```python
from build123d import *

# Parameters (mm, degrees)
SKETCH1_W           = 80
SKETCH1_H           = 40
BOSS_EXTRUDE1_DEPTH = 3
SKETCH2_R           = 2
SKETCH2_R_2         = 1
BOSS_EXTRUDE3_DEPTH = 10
LPATTERN1_COUNT     = 2
LPATTERN1_PITCH     = 20
SKETCH3_R           = 2
SKETCH3_R_2         = 1
BOSS_EXTRUDE4_DEPTH = 15
LPATTERN2_COUNT     = 2
LPATTERN2_PITCH     = 25


with BuildPart() as part:
    # Sketch1 → Boss-Extrude1 (new body)
    with BuildSketch(Plane.XY):
        Rectangle(SKETCH1_W, SKETCH1_H)
    extrude(amount=BOSS_EXTRUDE1_DEPTH)

    # Sketch2 → Boss-Extrude3 (add)
    with BuildSketch(Plane(origin=(0, 20, 0), x_dir=(1, 0, 0), z_dir=(0, 1, 0))):
        with Locations((-41.322875656, -1.5)):
            Circle(SKETCH2_R)
        with Locations(Location((-41.322875656, -1.5, 0), (0, 0, 270))):
            Circle(SKETCH2_R_2, mode=Mode.SUBTRACT)
    boss_extrude3 = extrude(amount=-BOSS_EXTRUDE3_DEPTH)

    # LPattern1: Boss-Extrude3 ×2
    with Locations(*[(0, -i * LPATTERN1_PITCH, 0) for i in range(1, LPATTERN1_COUNT)]):
        add(boss_extrude3)

    # Sketch3 → Boss-Extrude4 (add)
    with BuildSketch(Plane(origin=(0, 20, 0), x_dir=(1, 0, 0), z_dir=(0, 1, 0))):
        with Locations((41.322875656, -1.5)):
            Circle(SKETCH3_R)
        with Locations(Location((41.322875656, -1.5, 0), (0, 0, 270))):
            Circle(SKETCH3_R_2, mode=Mode.SUBTRACT)
    boss_extrude4 = extrude(amount=-BOSS_EXTRUDE4_DEPTH)

    # LPattern2: Boss-Extrude4 ×2
    with Locations(*[(0, -i * LPATTERN2_PITCH, 0) for i in range(1, LPATTERN2_COUNT)]):
        add(boss_extrude4)


solid = part.part
```
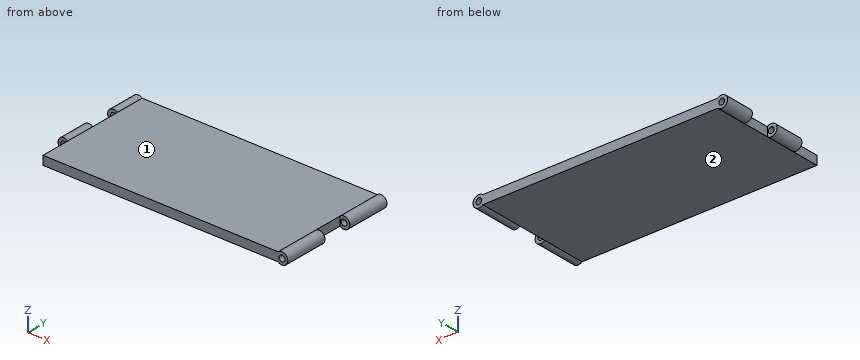
Geometry check sheet. Reference: the model listing, model coordinates, mm. Face numbers are marked on the shaded views. Give positions to 0.01 mm unless a question says otherwise; leave off trailing zeros. Write each loop counter-clockwise with the first axis right and the second up, starting at its lowest first coordinate (ties: lowest second). Pieces come first, ordered by that corner, then holes. Notation, with made-up numbers: (20.25, -36.5) -> (36.25, -36.5) arc R33 ccw to (36.25, -6.5) -> close; hole circle Ø6 at (42, 33.25). An arc over 180 degrees is marked (long way). One line per question, with ' | ' between items.
Item 1: Sectioned sample at C-C, the plane y = -16.5. Record the boundary of the cut face in (x, z), plus the area to 3 significant figures.
Determined:
outline: (-40, 0) -> (40, 0) arc R2 ccw (long way) to (40, 3) -> (-40, 3) -> close; hole circle Ø2 at (41.32, 1.5) | area: 248 mm^2
Item 2: Sectioned sample at A-A, the plane z = 1.5. State how many separate pieces and enclosed holes the cut face has, plus the area to 3 significant figures.
Determined:
separate pieces: 5 | enclosed holes: 0 | area: 3,270 mm^2
Item 3: Sectioned sample at B-B, the plane y = -7. Record the boundary of the cut face in (x, z), plus the area to 3 significant figures.
Determined:
outline: (-40, 0) -> (40, 0) arc R2 ccw (long way) to (40, 3) -> (-40, 3) arc R2 ccw (long way) to start; hole circle Ø2 at (-41.32, 1.5); hole circle Ø2 at (41.32, 1.5) | area: 256 mm^2
Item 4: Draft check along X on the marked faces 1 and 2. Enter one of: released by +X, released by -X, zero draft, split by the parting line, or undercut.
Determined:
face 1: undercut | face 2: undercut
Item 5: Sectioned sample at D-D, the plane x = 38.5. Record the boundary of the cut face in (y, z), plus the area to 3 significant figures.
Determined:
outline: (-20, 0) -> (20, 0) -> (20, 3) -> (-20, 3) -> close | area: 120 mm^2
Item 6: Scan lines: line 1 along X through (y, z) = (13.75, 1.5); line 2 along X through (y, z) = (-2.75, 1.5); line 3 along X through (y, z) = (-14.5, 1.5). Record each from-to range of solid material in increasing order.
Determined:
line 1: -43.32 to -42.32, -40.32 to 40.32, 42.32 to 43.32 | line 2: -43.32 to -42.32, -40.32 to 40 | line 3: -40 to 40.32, 42.32 to 43.32
Item 7: Depth check by flat-ended pin: pin 1 (1.5 mm diameter, centred on y = 4, z = 1, fed in from +X); pin 2 (20 mm diameter, centred on x = 9, y = -9.5, fed in from -Z); pin 3 (12 mm diameter, centred on x = 20.5, y = 5.5, fed in from +Z); pin 4 (1.8 mm diameter, centred on x = -41.32, z = 1.5, fed in from +Y). Enter the tip coordinate at first touch or a pass-through.
Determined:
pin 1: x = 40 | pin 2: z = 0 | pin 3: z = 3 | pin 4: through
